Build history of the part. All positions in model axes, mm. A direction names the side the tool comes from. Round coordinates to 2 decimals unless told otherwise and drop trailing zeros. Order: outer loops, then holes, each group sorted by start corner. A loop starts at its lowest first (then second) coordinate and runs counter-clockwise, first axis right, second up. Notation, with made-up numbers: M -38.5,-34 L -22.5,-34 A3 ccw -22.5,-30 Z; hole C 38,-24.5 d7. An arc over 180 degrees is marked long. One line per item, written item: value. Start each with the question number.
Item 1: Two-plate mould, pull along Z, no slides. Class faces 1 (the flat face through (17, 3, 123.952)), 2 (the cylindrical face through (-64.26, 1.79, 80.26)), 3 (the cylindrical face through (16.22, 9.74, 118.07)): +Z half, -Z half, draft (parallel to the pull), parting line (faces both ways), or undercut.
Item 2: Band-saw the part on C-C, the plane x = -30.5. Write the cut outline in (y, z).
Item 3: Band-saw the part on B-B, the plane y = -11.5. Write the cut outline in (x, z), then the cut area to 3 significant figures.
Item 4: Probe L1, parallel to Z at x = -16.5, y = -27; L2, parallel to X at y = -39, z = 42.5; L3, parallel to Y at x = -68.5, z = 115.5. List the from-to ranges inside material, lowest first.
Item 5: Pin check, flat tips, straight feed: pin 1 (3 mm diameter, centred on x = -23.5, z = 2, fed in from +Y); pin 2 (8 mm diameter, centred on x = -55, z = 23, fed in from -Y); pin 3 (3 mm diameter, centred on x = -11.5, y = -24.5, fed in from +Z); pin 4 (7 mm diameter, centred on x = -17, z = 2.5, fed in from -Y). Stop position of each tip, or through.
Item 6: Band-saw the part on D-D, the plane z = 77. Write the cut outline in (x, y).
Item 7: Band-saw the part on A-A, the plane z = 27.5. Write the cut outline in (x, y).
Item 8: Tool access for faces 4 (the conical face through (-70.517, 5.673, 108.463)), 5 (the cylindrical face through (21.47, -48.98, 3.13)), 6 (the cylindrical face through (16.4, -51.9, 118.1)), 7 (the cylindrical face through (-71.333, -48.885, 3.131)), 8 (the flat face through (-73.144, -20, 3)): list every direction of +Z, -Z, +X, -X, +Y, -Y with a clear straight run to the whole face (end or side of a thin tool).
```python
from build123d import *

# Parameters (mm, degrees)
F1_DEPTH     = 6.35
F2_R         = 5.9452870566
F3_DEPTH     = 46.736
F4_R         = 3.3233318127
F5_DEPTH     = 110.236
F7_START     = 108.204
F6_R         = 7.8492612618
F6_R_2       = 7.6458831821
F6_R_3       = 6.963642992
F6_R_4       = 6.7625316393
F7_DEPTH     = 15.748
F8_S9_R      = 3.3233318127
F8_T10_DEPTH = 11
F8_S15_R     = 3.3233318127
F8_T16_DEPTH = 12


# Not quite as in the source:
# - a fillet or chamfer that OpenCascade refuses, or shapes differently, is made with other operations: its cross-section is extruded or revolved along the edge and cut away or added


with BuildPart() as f1:
    # F0 (on Top) → F1 (new body)
    with BuildSketch(Plane.XY):
        with BuildLine():
            Line((17.025944097, 9.4035214942), (-66.794055903, 9.4035214942))
            ThreePointArc((-66.794055903, 9.4035214942), (-71.2841839635, 7.5436495547), (-73.144055903, 3.0535214942))
            Line((-73.144055903, 3.0535214942), (-73.144055903, -44.4444785058))
            ThreePointArc((-73.144055903, -44.4444785058), (-71.2841839635, -48.9346065664), (-66.794055903, -50.7944785058))
            Line((-66.794055903, -50.7944785058), (17.025944097, -50.7944785058))
            ThreePointArc((17.025944097, -50.7944785058), (21.5160721576, -48.9346065664), (23.375944097, -44.4444785058))
            Line((23.375944097, -44.4444785058), (23.375944097, 3.0535214942))
            ThreePointArc((23.375944097, 3.0535214942), (21.5160721576, 7.5436495547), (17.025944097, 9.4035214942))
        make_face()
    extrude(amount=F1_DEPTH)

    # F2 (on face) → F3 (join)
    with BuildSketch(Plane.XY.offset(6.35)):
        with Locations((-66.794055903, 3.0535214942)):
            Circle(F2_R)
        with Locations((17.025944097, 3.0535214942)):
            Circle(F2_R)
        with Locations((-66.794055903, -44.4444785058)):
            Circle(F2_R)
        with Locations((17.025944097, -44.4444785058)):
            Circle(F2_R)
    extrude(amount=F3_DEPTH)

    # F4 (on Top) → F5 (join)
    with BuildSketch(Plane.XY):
        with Locations((-67.3308223486, 3.0604917556)):
            Circle(F4_R)
        with Locations((16.9055722654, 3.0604917556)):
            Circle(F4_R)
        with Locations((-67.3308223486, -44.4500036538)):
            Circle(F4_R)
        with Locations((17.4885243177, -45.0329519808)):
            Circle(F4_R)
    extrude(amount=F5_DEPTH)

    # F6 (on Top) → F7 (join)
    with BuildSketch(Plane.XY.offset(F7_START)):
        with Locations((-67.5922632217, 2.9914693441)):
            Circle(F6_R)
        with Locations((-67.435964942, -44.5234365761)):
            Circle(F6_R_2)
        with Locations((17.121816054, 2.8351708315)):
            Circle(F6_R_3)
        with Locations((17.9033093154, -45.3049317002)):
            Circle(F6_R_4)
    extrude(amount=F7_DEPTH)

    # F8: chamfer of 4.1402 on 4 edges, made by hand

    # F8_s1 → F8_t2 (revolve, cut)
    with BuildSketch(Plane.XZ.offset(44.5234365761)):
        Polygon((-63.9302817599, 108.204), (-59.7900817599, 112.3442), (-59.7900817599, 108.204), align=None)
    revolve(axis=Axis((-67.435964942, -44.5234365761, 108.204), (0, 0, 1)), mode=Mode.SUBTRACT)

    # F8_s3 → F8_t4 (revolve, cut)
    with BuildSketch(Plane.XZ.offset(-2.9914693441)):
        Polygon((-63.8832019599, 108.204), (-59.7430019599, 112.3442), (-59.7430019599, 108.204), align=None)
    revolve(axis=Axis((-67.5922632217, 2.9914693441, 108.204), (0, 0, 1)), mode=Mode.SUBTRACT)


with BuildPart() as f8_tool6:
    # F8_s7 → F8_t8 (revolve)
    with BuildSketch(Plane.XZ.offset(45.3049317002)):
        Polygon((20.5256409548, 108.204), (24.6658409548, 112.3442), (24.6658409548, 108.204), align=None)
    revolve(axis=Axis((17.9033093154, -45.3049317002, 108.204), (0, 0, 1)))

    # F8_s9 → F8_t10 (cut, symmetric)
    with BuildSketch(Plane.XY.offset(110.3)):
        with Locations((17.4885243177, -45.0329519808)):
            Circle(F8_S9_R)
    extrude(amount=F8_T10_DEPTH, both=True, mode=Mode.SUBTRACT)


with BuildPart() as f1_1:
    add(f1.part)

    # F8_t5: cut F8_tool6
    add(f8_tool6.part, mode=Mode.SUBTRACT)


with BuildPart() as f8_tool12:
    # F8_s13 → F8_t14 (revolve)
    with BuildSketch(Plane.XZ.offset(-2.8351708315)):
        Polygon((19.945259046, 108.204), (24.085459046, 112.3442), (24.085459046, 108.204), align=None)
    revolve(axis=Axis((17.121816054, 2.8351708315, 108.204), (0, 0, 1)))

    # F8_s15 → F8_t16 (cut, symmetric)
    with BuildSketch(Plane.XY.offset(110.3)):
        with Locations((16.9055722654, 3.0604917556)):
            Circle(F8_S15_R)
    extrude(amount=F8_T16_DEPTH, both=True, mode=Mode.SUBTRACT)


with BuildPart() as f1_2:
    add(f1_1.part)

    # F8_t11: cut F8_tool12
    add(f8_tool12.part, mode=Mode.SUBTRACT)


solid = f1_2.part
```
Output:
1. face 1: +Z half
1. face 2: undercut
1. face 3: draft
2. outline: M -50.79,0 L 9.4,0 L 9.4,6.35 L -50.79,6.35 Z
3. outline: M -73.14,0 L 23.38,0 L 23.38,6.35 L -73.14,6.35 Z
3. area: 613 mm²
4. L1: z = 0 to 6.35
4. L2: x = -69.18 to -64.41, 14.64 to 19.41
4. L3: y = -52.09 to -36.95, -4.81 to 10.79
5. pin 1: stops at y = 9.4
5. pin 2: passes through
5. pin 3: stops at z = 6.35
5. pin 4: stops at y = -50.79
6. outline: C -67.33,-44.45 d6.65; C -67.33,3.06 d6.65; C 16.91,3.06 d6.65; C 17.49,-45.03 d6.65
7. outline: C -66.79,-44.44 d11.89; C -66.79,3.05 d11.89; C 17.03,-44.44 d11.89; C 17.03,3.05 d11.89
8. face 4: none
8. face 5: -Z, +X, -Y
8. face 6: +Z
8. face 7: -Z, -X, -Y
8. face 8: -Z, -X, +Y, -Y
